Input: dimensioned drawing with shaded views. Units: mm. Origin: part minimum x, y, z. A direction names the side the tool comes from. Give positions to 0.01 mm unless a question says otherwise; leave off trailing zeros. Write each loop counter-clockwise with the first axis right and the second up, starting at its lowest first coordinate (ties: lowest second). Pieces come first, ordered by that corner, then holes.
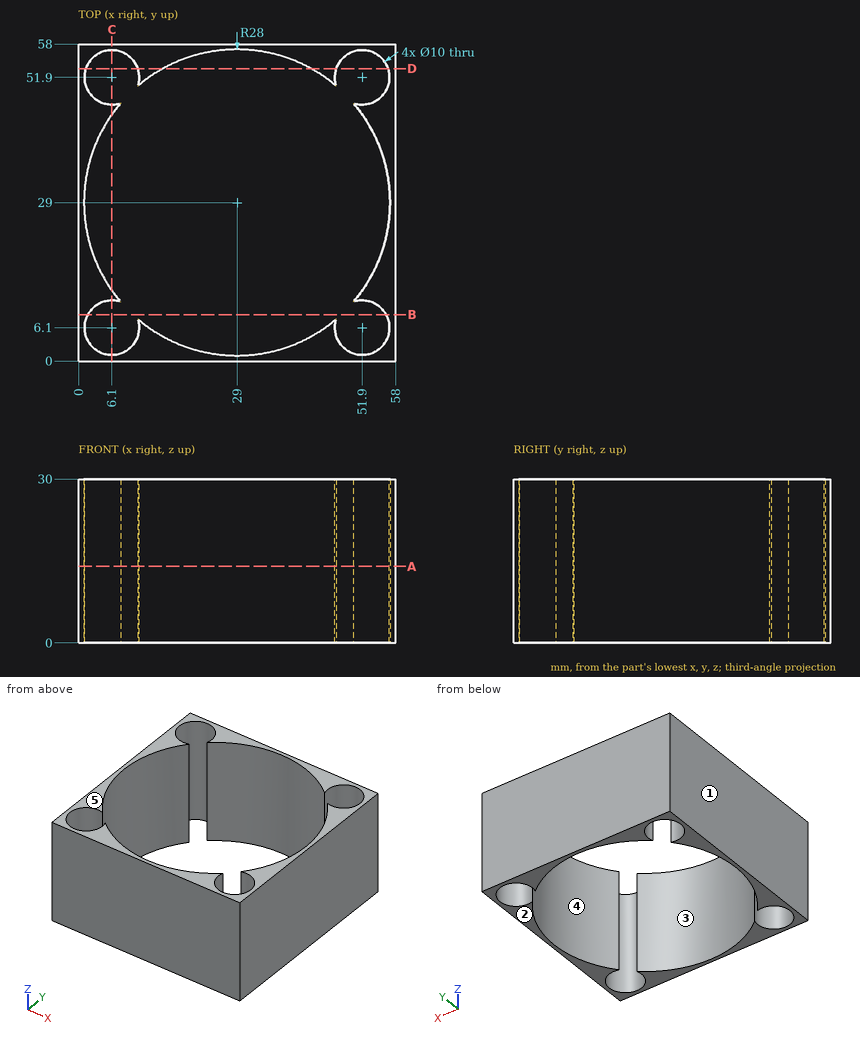
1. Cut plane C-C, the plane x = 6.1. Return the cut outline in (y, z).
2. Cut plane D-D, the plane y = 53.5. Return the cut outline in (x, z), then the cut area to 3 significant figures.
3. Contact query for a flat-ended pin moving along its axis: P1, Ø9, axis at x = 6.1, y = 6.1, coming from the +Z side. Output: stop coordinate, or through.
4. Access query for the marked faces 4 and 5. Directions: +Z, -Z, +X, -X, +Y, -Y. A direction counts if a zero-diameter tool reaches every point of the face in a straight line with its end or side. Return the directions, or none.
5. Cut plane B-B, the plane y = 8.5. Return the cut outline in (x, z), then the cut area to 3 significant figures.
6. Mould query, pull axis X, two halves, no side actions, for the marked faces 1, 2 and 3. Classes: +X half, -X half, draft (parallel to the pull), parting line (faces both ways), or undercut.
7. Cut plane A-A, the plane z = 14. Return the cut outline in (x, y).
8. Line query: L1, parallel to Y at x = 51.9, z = 21.75; L2, parallel to X at y = 7, z = 8.75. Output: solid intervals per line, ascending.
Response values:
1. outline: (0, 0) - (1.1, 0) - (1.1, 30) - (0, 30) - close; (11.1, 0) - (12.89, 0) - (12.89, 30) - (11.1, 30) - close; (45.11, 0) - (46.9, 0) - (46.9, 30) - (45.11, 30) - close; (56.9, 0) - (58, 0) - (58, 30) - (56.9, 30) - close
2. outline: (0, 0) - (1.36, 0) - (1.36, 30) - (0, 30) - close; (10.84, 0) - (15.44, 0) - (15.44, 30) - (10.84, 30) - close; (42.56, 0) - (47.16, 0) - (47.16, 30) - (42.56, 30) - close; (56.64, 0) - (58, 0) - (58, 30) - (56.64, 30) - close
2. area: 358 mm2
3. P1: passes through
4. face 4: +Z, -Z
4. face 5: +Z, +X, -X, +Y, -Y
5. outline: (0, 0) - (1.71, 0) - (1.71, 30) - (0, 30) - close; (56.29, 0) - (58, 0) - (58, 30) - (56.29, 30) - close
5. area: 103 mm2
6. face 1: -X half
6. face 2: draft
6. face 3: undercut
7. outline: (0, 0) - (58, 0) - (58, 58) - (0, 58) - close; hole (7.69, 10.84) arc R5 ccw (long way) to (10.84, 7.69) arc R28 ccw to (47.16, 7.69) arc R5 ccw (long way) to (50.31, 10.84) arc R28 ccw to (50.31, 47.16) arc R5 ccw (long way) to (47.16, 50.31) arc R28 ccw to (10.84, 50.31) arc R5 ccw (long way) to (7.69, 47.16) arc R28 ccw to start
8. L1: y = 0 to 1.1, 11.1 to 12.89, 45.11 to 46.9, 56.9 to 58
8. L2: x = 0 to 1.18, 11.02 to 11.68, 46.32 to 46.98, 56.82 to 58
